from build123d import *

# Parameters (mm, degrees)
BOSS_EXTRUDE1_DEPTH = 25
MOUNT_HOLES_DEPTH   = 41.422765863
SKETCH7_W           = 16.5
SKETCH7_H           = 26
CUT_PART_DEPTH      = 20
AXIS_R              = 2.75
CUT_EXTRUDE3_DEPTH  = 30
CUT_EXTRUDE4_DEPTH  = 1.5
CUT_EXTRUDE5_DEPTH  = 2
CHAMFER2_SIZE       = 2


with BuildPart() as part:
    # contour → Boss-Extrude1 (new, symmetric)
    with BuildSketch(Plane.XY):
        with BuildLine():
            Line((7.5, 0), (7.721344931, -6.500579199))
            Line((7.721344931, -6.500579199), (6.755375242, -7.5))
            Line((6.755375242, -7.5), (0, -7.5))
            Line((0, -7.5), (-28, -7.5))
            Line((-28, -7.5), (-28, -7.827e-05))
            Line((-28, -7.827e-05), (-7.5, -7.827e-05))
            ThreePointArc((-7.5, -7.827e-05), (-3.9135e-05, 7.5), (7.5, 0))
        make_face()
    extrude(amount=BOSS_EXTRUDE1_DEPTH, both=True)

    # Sketch6 → mount-holes (cut, through all)
    with BuildSketch(Plane.XZ.offset(7.5)):
        with BuildLine():
            Line((-21, 15.25), (-17, 15.25))
            ThreePointArc((-17, 15.25), (-14.25, 12.5), (-17, 9.75))
            Line((-17, 9.75), (-21, 9.75))
            ThreePointArc((-21, 9.75), (-23.75, 12.5), (-21, 15.25))
        make_face()
        with BuildLine():
            Line((-21, -9.75), (-17, -9.75))
            ThreePointArc((-17, -9.75), (-14.25, -12.5), (-17, -15.25))
            Line((-17, -15.25), (-21, -15.25))
            ThreePointArc((-21, -15.25), (-23.75, -12.5), (-21, -9.75))
        make_face()
    extrude(amount=-MOUNT_HOLES_DEPTH, mode=Mode.SUBTRACT)

    # Sketch7 → cut-part (cut)
    with BuildSketch(Plane.XZ.offset(7.5)):
        with Locations((-0.528655069, 0)):
            Rectangle(SKETCH7_W, SKETCH7_H)
    extrude(amount=-CUT_PART_DEPTH, mode=Mode.SUBTRACT)

    # axis → Cut-Extrude3 (cut, symmetric)
    with BuildSketch(Plane.XY):
        Circle(AXIS_R)
    extrude(amount=CUT_EXTRUDE3_DEPTH, both=True, mode=Mode.SUBTRACT)

    # Sketch9 → Cut-Extrude4 (cut)
    with BuildSketch(Plane.XZ.offset(7.5)):
        with BuildLine():
            Line((-17, 18.75), (-21, 18.75))
            ThreePointArc((-21, 18.75), (-27.25, 12.5), (-21, 6.25))
            Line((-21, 6.25), (-17, 6.25))
            ThreePointArc((-17, 6.25), (-10.75, 12.5), (-17, 18.75))
        make_face()
        with BuildLine():
            Line((-21, -18.75), (-17, -18.75))
            ThreePointArc((-17, -18.75), (-10.75, -12.5), (-17, -6.25))
            Line((-17, -6.25), (-21, -6.25))
            ThreePointArc((-21, -6.25), (-27.25, -12.5), (-21, -18.75))
        make_face()
    extrude(amount=-CUT_EXTRUDE4_DEPTH, mode=Mode.SUBTRACT)

    # Chamfer1
    # the kernel refuses this chamfer: 2 mm, written as the material it takes off along each edge
    with BuildSketch(Plane(origin=(7.324969659, 5.140386945, -25), x_dir=(0.027479951033163995, 0.0009356932186842305, 0.9996219169112968), z_dir=(0.03403031050568426, -0.9994208012478462, 0))) as chamfer1_piece_1_section:
        with BuildLine():
            Line((2.05734639, 0), (-0.11309431, 2.054235587))
            Line((-0.11309431, 2.054235587), (-0.153079186, 2.053135752))
            ThreePointArc((-0.153079186, 2.053135752), (-0.068258454, 1.026795659), (-0.039984877, -0.001099835))
            Line((-0.039984877, -0.001099835), (0.001099835, -0.039984877))
            ThreePointArc((0.001099835, -0.039984877), (1.028995329, -0.011711299), (2.058446225, -0.039984877))
            Line((2.058446225, -0.039984877), (2.05734639, 0))
        make_face()
    chamfer1_piece_1 = extrude(amount=16.79107846, mode=Mode.PRIVATE)
    chamfer1_piece_1 = split(chamfer1_piece_1, bisect_by=Plane(origin=(7.719880972, -6.502093854, -23.313005801), z_dir=(-0.7190376591339585, 0.6949711107284657, 0)), keep=Keep.TOP, mode=Mode.PRIVATE)
    add(chamfer1_piece_1, mode=Mode.SUBTRACT)
    with BuildSketch(Plane(origin=(7.324969659, 5.140386945, 25), x_dir=(-0.9990429371443961, -0.03401744422077874, 0.027495876610585647), z_dir=(0.03403031050568426, -0.9994208012478462, 0))) as chamfer1_piece_2_section:
        with BuildLine():
            Line((2.05734639, 0), (-0.11309431, 2.054235587))
            Line((-0.11309431, 2.054235587), (-0.153079186, 2.053135752))
            ThreePointArc((-0.153079186, 2.053135752), (-0.068258454, 1.026795659), (-0.039984877, -0.001099835))
            Line((-0.039984877, -0.001099835), (0.001099835, -0.039984877))
            ThreePointArc((0.001099835, -0.039984877), (1.028995329, -0.011711299), (2.058446225, -0.039984877))
            Line((2.058446225, -0.039984877), (2.05734639, 0))
        make_face()
    chamfer1_piece_2 = extrude(amount=16.79107846, mode=Mode.PRIVATE)
    chamfer1_piece_2 = split(chamfer1_piece_2, bisect_by=Plane(origin=(10.54505629, -3.579083939, 24.461957422), z_dir=(-0.7190376591339585, 0.6949711107284657, 0)), keep=Keep.TOP, mode=Mode.PRIVATE)
    add(chamfer1_piece_2, mode=Mode.SUBTRACT)
    with BuildSketch(Plane(origin=(-28, -7.5, -25), x_dir=(0.9996219169112968, 0, -0.027495876610585647), z_dir=(0, 1, 0)), Plane(origin=(-28, -7.5, 25), x_dir=(-0.027495876610585647, 0, -0.9996219169112968), z_dir=(0, 1, 0))) as chamfer1_piece_3:
        with BuildLine():
            Line((2.05734639, 0), (-0.11309431, -2.054235587))
            Line((-0.11309431, -2.054235587), (-0.153079186, -2.053135752))
            ThreePointArc((-0.153079186, -2.053135752), (-0.068258454, -1.026795659), (-0.039984877, 0.001099835))
            Line((-0.039984877, 0.001099835), (0.001099835, 0.039984877))
            ThreePointArc((0.001099835, 0.039984877), (1.028995329, 0.011711299), (2.058446225, 0.039984877))
            Line((2.058446225, 0.039984877), (2.05734639, 0))
        make_face()
    extrude(amount=7.49992173, mode=Mode.SUBTRACT)
    with BuildSketch(Plane(origin=(0, 0, -25), x_dir=(-0.7732184624570568, -0.6341397395807529, 0), z_dir=(0.6341397395807529, -0.7732184624570568, 0))) as chamfer1_piece_4_section:
        with BuildLine():
            Line((7.556568542, -2.056568542), (5.443431458, 0.056568542))
            Line((5.443431458, 0.056568542), (5.443431458, 0.096568542))
            ThreePointArc((5.443431458, 0.096568542), (6.471715729, 0.04), (7.5, 0.04))
            Line((7.5, 0.04), (7.54, 0))
            ThreePointArc((7.54, 0), (7.54, -1.028284271), (7.596568542, -2.056568542))
            Line((7.596568542, -2.056568542), (7.556568542, -2.056568542))
        make_face()
    chamfer1_piece_4 = revolve(axis=Axis((0, 0, -25), (0, 0, -1)), revolution_arc=258.711821509, mode=Mode.PRIVATE)
    chamfer1_piece_4 = split(chamfer1_piece_4, bisect_by=Plane(origin=(0, -7.827e-05, -24.025554596), z_dir=(0, 1, 0)), keep=Keep.TOP, mode=Mode.PRIVATE)
    chamfer1_piece_4 = split(chamfer1_piece_4, bisect_by=Plane(origin=(7.269376506, 6.773077101, -24.025554596), z_dir=(-0.9994208012478462, -0.03403031050568426, 0)), keep=Keep.TOP, mode=Mode.PRIVATE)
    add(chamfer1_piece_4, mode=Mode.SUBTRACT)
    with BuildSketch(Plane(origin=(0, 0, 25), x_dir=(-0.7732184624570568, -0.6341397395807529, 0), z_dir=(0.6341397395807529, -0.7732184624570568, 0))) as chamfer1_piece_5_section:
        with BuildLine():
            Line((5.443431458, -0.056568542), (7.556568542, 2.056568542))
            Line((7.556568542, 2.056568542), (7.596568542, 2.056568542))
            ThreePointArc((7.596568542, 2.056568542), (7.54, 1.028284271), (7.54, 0))
            Line((7.54, 0), (7.5, -0.04))
            ThreePointArc((7.5, -0.04), (6.471715729, -0.04), (5.443431458, -0.096568542))
            Line((5.443431458, -0.096568542), (5.443431458, -0.056568542))
        make_face()
    chamfer1_piece_5 = revolve(axis=Axis((0, 0, 25), (0, 0, -1)), revolution_arc=258.711821509, mode=Mode.PRIVATE)
    chamfer1_piece_5 = split(chamfer1_piece_5, bisect_by=Plane(origin=(0, -7.827e-05, 24.025554599), z_dir=(0, 1, 0)), keep=Keep.TOP, mode=Mode.PRIVATE)
    chamfer1_piece_5 = split(chamfer1_piece_5, bisect_by=Plane(origin=(7.269376506, 6.773077103, 24.025554599), z_dir=(-0.9994208012478462, -0.03403031050568426, 0)), keep=Keep.TOP, mode=Mode.PRIVATE)
    add(chamfer1_piece_5, mode=Mode.SUBTRACT)

    # Sketch10 → Cut-Extrude5 (cut)
    with BuildSketch(Plane(origin=(0, -7.827e-05, 0), x_dir=(1, 0, 0), z_dir=(0, 1, 0))):
        Polygon((-11.278655069, 4), (-25, 4), (-25, 21.757359313), (-24.757359313, 22), (-12.278655069, 22), (-11.278655069, 21), align=None)
        Polygon((-11.278655069, -4), (-25, -4), (-25, -21.757359313), (-24.757359313, -22), (-12.278655069, -22), (-11.278655069, -21), align=None)
    extrude(amount=-CUT_EXTRUDE5_DEPTH, mode=Mode.SUBTRACT)

    # Chamfer2
    # the kernel refuses this chamfer: 2 mm, written as the material it adds along each edge
    with BuildSketch(Plane(origin=(-29.900725289, -2.00007827, 22), x_dir=(0, 0.9996219169112968, 0.02749587661058563), z_dir=(1, 0, 0))) as chamfer2_piece_1_section:
        Polygon((CHAMFER2_SIZE * 0.999621916911, -CHAMFER2_SIZE * 0.0274958766106), (-CHAMFER2_SIZE * 0.0274958766106, -CHAMFER2_SIZE * 0.999621916911), (0, 0), align=None)
    chamfer2_piece_1 = extrude(amount=22.765436196, mode=Mode.PRIVATE)
    chamfer2_piece_1 = split(chamfer2_piece_1, bisect_by=Plane(origin=(-25, -1.339790295, 21.320575951), z_dir=(1, 0, 0)), keep=Keep.TOP, mode=Mode.PRIVATE)
    add(chamfer2_piece_1)
    with BuildSketch(Plane(origin=(-25, -2.00007827, 1.143365976), x_dir=(-0.02749587661058563, 0.9996219169112968, 0), z_dir=(0, 0, -1))) as chamfer2_piece_2_section:
        Polygon((CHAMFER2_SIZE * 0.999621916911, CHAMFER2_SIZE * 0.0274958766106), (-CHAMFER2_SIZE * 0.0274958766106, CHAMFER2_SIZE * 0.999621916911), (0, 0), align=None)
    chamfer2_piece_2 = extrude(amount=28.044091265, mode=Mode.PRIVATE)
    chamfer2_piece_2 = split(chamfer2_piece_2, bisect_by=Plane(origin=(-24.347473985, -1.326341277, -22), z_dir=(0, 0, 1)), keep=Keep.TOP, mode=Mode.PRIVATE)
    chamfer2_piece_2 = chamfer2_piece_2 - Plane(origin=(-21, -1.326341277, -12.5), x_dir=(0, 0, -1), z_dir=(0, -1, 0)) * Cylinder(2.75, 65, mode=Mode.PRIVATE)
    add(chamfer2_piece_2)
    with BuildSketch(Plane(origin=(-29.900725289, -2.00007827, -22), x_dir=(1.7831818563715163e-15, 0.9996219169112968, -0.02749587661058563), z_dir=(1, 0, 0))) as chamfer2_piece_3_section:
        Polygon((CHAMFER2_SIZE * 0.999621916911, CHAMFER2_SIZE * 0.0274958766106), (-CHAMFER2_SIZE * 0.0274958766106, CHAMFER2_SIZE * 0.999621916911), (0, 0), align=None)
    chamfer2_piece_3 = extrude(amount=22.765436196, mode=Mode.PRIVATE)
    chamfer2_piece_3 = split(chamfer2_piece_3, bisect_by=Plane(origin=(-21.883009307, -1.339790295, -24.874350006), z_dir=(0.7071067811864957, 0, 0.7071067811865993)), keep=Keep.TOP, mode=Mode.PRIVATE)
    add(chamfer2_piece_3)
    with BuildSketch(Plane(origin=(-11.278655069, -2.00007827, -26.143365976), x_dir=(0.027495876610586494, 0.9996219169112968, 0), z_dir=(0, 0, 1))) as chamfer2_piece_4_section:
        Polygon((CHAMFER2_SIZE * 0.999621916911, CHAMFER2_SIZE * 0.0274958766106), (-CHAMFER2_SIZE * 0.0274958766106, CHAMFER2_SIZE * 0.999621916911), (0, 0), align=None)
    chamfer2_piece_4 = extrude(amount=27.286731952, mode=Mode.PRIVATE)
    chamfer2_piece_4 = split(chamfer2_piece_4, bisect_by=Plane(origin=(-7.513844642, -1.337755995, -17.235189573), z_dir=(-0.707106781186572, 0, 0.707106781186523)), keep=Keep.TOP, mode=Mode.PRIVATE)
    add(chamfer2_piece_4)
    with BuildSketch(Plane(origin=(-11.278655069, -2.00007827, -4), x_dir=(0, 0.9996219169112968, 0.027495876610586275), z_dir=(-1, 0, 0))) as chamfer2_piece_5:
        Polygon((CHAMFER2_SIZE * 0.999621916911, CHAMFER2_SIZE * 0.0274958766106), (-CHAMFER2_SIZE * 0.0274958766106, CHAMFER2_SIZE * 0.999621916911), (0, 0), align=None)
    extrude(amount=13.721344931)
    with BuildSketch(Plane(origin=(-25, -2.00007827, -1.143365976), x_dir=(-0.02749587661058563, 0.9996219169112968, 0), z_dir=(0, 0, 1))) as chamfer2_piece_6_section:
        Polygon((CHAMFER2_SIZE * 0.999621916911, -CHAMFER2_SIZE * 0.0274958766106), (-CHAMFER2_SIZE * 0.0274958766106, -CHAMFER2_SIZE * 0.999621916911), (0, 0), align=None)
    chamfer2_piece_6 = extrude(amount=28.044091265, mode=Mode.PRIVATE)
    chamfer2_piece_6 = split(chamfer2_piece_6, bisect_by=Plane(origin=(-29.055362029, -1.326341277, 17.701997284), z_dir=(0.7071067811865476, 0, -0.7071067811865476)), keep=Keep.TOP, mode=Mode.PRIVATE)
    chamfer2_piece_6 = chamfer2_piece_6 - Plane(origin=(-21, -1.326341277, 12.5), x_dir=(0, 0, -1), z_dir=(0, -1, 0)) * Cylinder(2.75, 65, mode=Mode.PRIVATE)
    add(chamfer2_piece_6)
    with BuildSketch(Plane(origin=(-11.278655069, -2.00007827, 4), x_dir=(0, 0.9996219169112968, -0.027495876610586275), z_dir=(-1, 0, 0))) as chamfer2_piece_7:
        Polygon((CHAMFER2_SIZE * 0.999621916911, -CHAMFER2_SIZE * 0.0274958766106), (-CHAMFER2_SIZE * 0.0274958766106, -CHAMFER2_SIZE * 0.999621916911), (0, 0), align=None)
    extrude(amount=13.721344931)
    with BuildSketch(Plane(origin=(-11.278655069, -2.00007827, 26.143365976), x_dir=(0.027495876610586494, 0.9996219169112968, 0), z_dir=(0, 0, -1))) as chamfer2_piece_8_section:
        Polygon((CHAMFER2_SIZE * 0.999621916911, -CHAMFER2_SIZE * 0.0274958766106), (-CHAMFER2_SIZE * 0.0274958766106, -CHAMFER2_SIZE * 0.999621916911), (0, 0), align=None)
    chamfer2_piece_8 = extrude(amount=27.286731952, mode=Mode.PRIVATE)
    chamfer2_piece_8 = split(chamfer2_piece_8, bisect_by=Plane(origin=(-11.954010519, -1.337755995, 22), z_dir=(0, 0, -1)), keep=Keep.TOP, mode=Mode.PRIVATE)
    add(chamfer2_piece_8)


solid = part.part
Geometry: final body of the model. Coordinates: model frame, mm. A direction names the side the tool comes from. Give positions to 0.01 mm unless a question says otherwise; leave off trailing zeros. Order: outer loops, then holes, each group sorted by start corner. A loop starts at its lowest first (then second) coordinate and runs counter-clockwise, first axis right, second up. Notation, with made-up numbers: (-9.75, -5.5) -> (21.25, -5.5) arc R25 ccw to (21.25, 10.5) -> close; hole circle Ø3 at (69.25, 58). An arc over 180 degrees is marked (long way). Answer as a JSON object with one key per item and string values.
Q1. Access query for faces 1 (the flat face through (-18, -2, -16)), 2 (the cylindrical face through (-10.75, -6.76, -12.64)), 3 (the cylindrical face through (-23.75, -4.14, 12.56)). Directions: +Z, -Z, +X, -X, +Y, -Y. A direction counts if a zero-diameter tool reaches every point of the face in a straight line with its end or side. Return the directions, or none.
Entries:
{"face 1": "+Y", "face 2": "-Y", "face 3": "+Y, -Y"}
Q2. Draft query along Y for faces 4 (the cylindrical face through (-10.75, -6.76, 12.36)), 5 (the flat face through (-19.1, -6, -9.6)), 6 (the flat face through (-18, -1, -5)), 7 (the cylindrical face through (-0.596, -2.685, -18.916)). Return one class per face: released by +Y, released by -Y, zero draft, split by the parting line, or undercut.
Entries:
{"face 4": "zero draft", "face 5": "released by -Y", "face 6": "released by +Y", "face 7": "undercut"}
Q3. Section C-C (z = -0.5). Output: boundary loops of the cut face in (x, y).
Entries:
{"outline": "(-28, -7.5) -> (-8.78, -7.5) -> (-8.78, 0) -> (-28, 0) -> close"}
Q4. Material intervals for probe 1 along Z at (x, y) = (-20.5, -6.5); probe 2 along Y at (x, z) = (0, -16.5); probe 3 along Z at (x, y) = (-8.5, -3), sorted ascending.
Entries:
{"probe 1": "z = -25 to -18.75, -6.25 to 6.25, 18.75 to 25", "probe 2": "y = -7.5 to -2.75, 2.75 to 7.5", "probe 3": "z = -25 to -13, 13 to 25"}
Q5. Section B-B (z = -7.5). Output: boundary loops of the cut face in (x, y).
Entries:
{"outline": "(-28, -7.5) -> (-24.75, -7.5) -> (-24.75, -6) -> (-13.25, -6) -> (-13.25, -7.5) -> (-8.78, -7.5) -> (-8.78, 0) -> (-11.28, 0) -> (-13.28, -2) -> (-23, -2) -> (-25, 0) -> (-28, 0) -> close"}
Q6. First-contact query: pin 1 (1 mm diameter, centred on y = 1.5, z = -13.5, fed in from -X); pin 2 (3 mm diameter, centred on x = -5.5, z = -8, fed in from +Y); pin 3 (4 mm diameter, centred on x = -16.5, z = -14, fed in from -Y); pin 4 (8 mm diameter, centred on x = -18, z = -15, fed in from +Y). Flat tips, straight axial feed; report the tip coordinate or a pass-through.
Entries:
{"pin 1": "stops at x = -7.43", "pin 2": "passes through", "pin 3": "stops at y = -6", "pin 4": "stops at y = -2"}
Q7. Section A-A (x = 0). Output: boundary loops of the cut face in (y, z), plus the area to 3 significant figures.
Entries:
{"outline": "(-7.5, -25) -> (-2.75, -25) -> (-2.75, -13) -> (-7.5, -13) -> close; (-7.5, 13) -> (-2.75, 13) -> (-2.75, 25) -> (-7.5, 25) -> close; (2.75, -25) -> (5.5, -25) -> (7.5, -23) -> (7.5, -13) -> (2.75, -13) -> close; (2.75, 13) -> (7.5, 13) -> (7.5, 23) -> (5.5, 25) -> (2.75, 25) -> close", "area": "224 mm^2"}
